```python
from build123d import *

# Parameters (mm, degrees)
F0_W     = 20
F0_H     = 20
F0_R     = 2.2
F1_DEPTH = 7
F2_W     = 20
F2_H     = 7
F3_DEPTH = 27
F4_R     = 1.7
F5_DEPTH = 7
F6_R     = 5
F7_R     = 2


with BuildPart() as f1:
    # F0 (on Top) → F1 (new body)
    with BuildSketch(Plane.XY):
        with Locations((10, 10)):
            Rectangle(F0_W, F0_H)
        with Locations((10, 13.5)):
            Circle(F0_R, mode=Mode.SUBTRACT)
    extrude(amount=F1_DEPTH)

    # F2 (on Top) → F3 (join)
    with BuildSketch(Plane.XY):
        with Locations((10, 3.5)):
            Rectangle(F2_W, F2_H)
    extrude(amount=F3_DEPTH)

    # F4 (on face) → F5 (cut, through all)
    with BuildSketch(Plane.XZ):
        with Locations((2.7, 23.3)):
            Circle(F4_R)
        with Locations((16.7, 23.3)):
            Circle(F4_R)
    extrude(amount=-F5_DEPTH, mode=Mode.SUBTRACT)

    # F6
    f6_edges = [f1.edges().sort_by_distance(p)[0] for p in [
        (0, 20, 3.5),
        (20, 20, 3.5),
    ]]
    fillet(f6_edges, radius=F6_R)

    # F7
    f7_edges = [f1.edges().sort_by_distance(p)[0] for p in [
        (0, 3.5, 27),
        (20, 3.5, 27),
        (10, 7, 7),
    ]]
    fillet(f7_edges, radius=F7_R)


solid = f1.part
```
Check sheet for the modelled part. Datum: model origin and axes. Units: mm. A direction names the side the tool comes from. Coordinates: 2 decimals unless noted, no trailing zeros. Order: outer loops, then holes, each group sorted by start corner. A loop starts at its lowest first (then second) coordinate and runs counter-clockwise, first axis right, second up. Notation, with made-up numbers: M 19,14.25 L 70,14.25 A8 ccw 70,20.25 Z; hole C 29.5,85.25 d2. An arc over 180 degrees is marked long. One line per question, with ' | ' between items. Start each with the question number.
Item 1: Gauge pin test, flat ends, axial feed: P1, Ø9, axis at x = 8, z = 22, coming from the +Y side; P2, Ø9, axis at x = 11, y = 16.5, coming from the +Z side; P3, Ø10, axis at x = 5, z = 12.5, coming from the +Y side. Record the tip position at first contact, or that the pin passes through.
Item 2: Sectioned sample at B-B on x = 10. Record the cut outline in (y, z), and give its area (3 significant figures).
Item 3: Access from +Z, -Z, +X, -X, +Y, -Y to the whole of each face (thin tool, end or side, straight path). Record for faces 4 (the flat face through (10, 10, 0)), 5 (the flat face through (10, 7, 18)).
Item 4: Sectioned sample at A-A on y = 13.5. Record the cut outline in (x, z).
Item 5: Sectioned sample at D-D on z = 6.25. Record the cut outline in (x, y).
Item 6: Sectioned sample at C-C on z = 23.3. Record the cut outline in (x, y).
Item 7: Mould release check, pull along Y, two halves, no side actions. Record for faces 1 (the cylindrical face through (8.38, 14.99, 3.45)), 2 (the flat face through (10, 0, 13)), 3 (the flat face through (10, 16, 7)): pulls with the +Y half, pulls with the -Y half, needs draft (parallel to the pull), parting line crosses it, or undercut.
Item 8: Material ranges on line 1 (Z direction, x = 2.7, y = 4.25); line 2 (Y direction, x = 10, z = 4.5); line 3 (Z direction, x = 15.5, y = 5.5), recorded low to high.
Answer below:
1) P1: stops at y = 7 | P2: stops at z = 7 | P3: stops at y = 7.68
2) outline: M 0,0 L 11.3,0 L 11.3,7 L 9,7 A2 cw 7,9 L 7,27 L 0,27 Z; M 15.7,0 L 20,0 L 20,7 L 15.7,7 Z | area: 250 mm^2
3) face 4: -Z, +X, -X, +Y, -Y | face 5: +Z, +X, -X, +Y
4) outline: M 0,0 L 7.8,0 L 7.8,7 L 0,7 Z; M 12.2,0 L 20,0 L 20,7 L 12.2,7 Z
5) outline: M 0,0 L 20,0 L 20,15 A5 ccw 15,20 L 5,20 A5 ccw 0,15 Z; hole C 10,13.5 d4.4
6) outline: M 0,0 L 1,0 L 1,7 L 0,7 Z; M 4.4,0 L 15,0 L 15,7 L 4.4,7 Z; M 18.4,0 L 20,0 L 20,7 L 18.4,7 Z
7) face 1: undercut | face 2: pulls with the -Y half | face 3: needs draft
8) line 1: z = 0 to 21.6, 25 to 27 | line 2: y = 0 to 11.3, 15.7 to 20 | line 3: z = 0 to 22.1, 24.5 to 27
